from build123d import *

# Parameters (mm, degrees)
F0_R     = 8.5
F0_R_2   = 6.6901913145
F1_DEPTH = 25


# Not quite as in the source:
# - a feature names something its author has since deleted; it is built from what else it names


with BuildPart() as f1:
    # F0 (on Top) → F1 (new body)
    with BuildSketch(Plane.XY):
        with BuildLine():
            Line((147.8986507368, 41.0247598798), (-12.1013492632, 41.0247598798))
            ThreePointArc((-12.1013492632, 41.0247598798), (-33.5643369753, 37.6297800364), (-12.1013492632, 34.2348001929))
            Line((-12.1013492632, 34.2348001929), (-12.1013492632, 35.5247598798))
            Line((-12.1013492632, 35.5247598798), (147.8986507368, 35.5247598798))
            ThreePointArc((147.8986507368, 35.5247598798), (164.0425617184, 38.1300025139), (147.8986507368, 40.735245148))
            Line((147.8986507368, 40.735245148), (147.8986507368, 41.0247598798))
        make_face()
        with Locations((-22.5643369753, 37.6297800364)):
            Circle(F0_R, mode=Mode.SUBTRACT)
        with Locations((155.7603941795, 38.1300025139)):
            Circle(F0_R_2, mode=Mode.SUBTRACT)
    extrude(amount=F1_DEPTH)


solid = f1.part
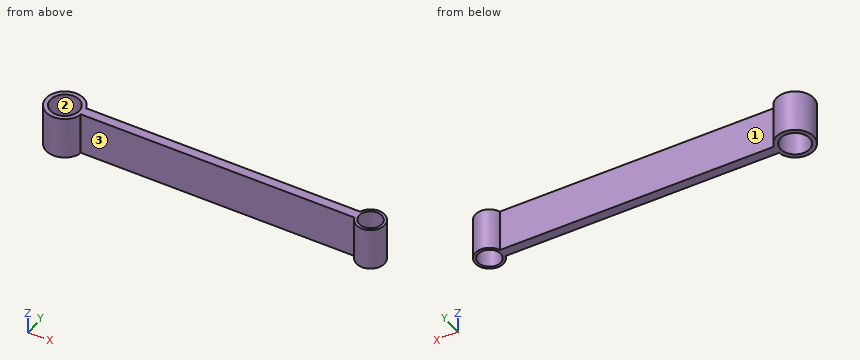
Build history of the part. All positions in model axes, mm. Face numbers are marked on the shaded views. A direction names the side the tool comes from. Coordinates: 2 decimals unless noted, no trailing zeros. Write each loop counter-clockwise with the first axis right and the second up, starting at its lowest first coordinate (ties: lowest second). Pieces come first, ordered by that corner, then holes.
(1) Pin check, flat tips, straight feed: pin 1 Ø7.5 at (x, z) = (63, 9) entering from +Y; pin 2 Ø4 at (x, z) = (-12, 3) entering from +Y; pin 3 Ø6 at (y, z) = (44, 11) entering from -X. Stop position of each tip, or through.
(2) Drill centre lines: line 1 (Y direction, x = 156, z = 17.75); line 2 (X direction, y = 36, z = 4.5); line 3 (X direction, y = 33.5, z = 4) (3 decimals). Where is each one in solid material? Low to high.
(3) 3-axis set-ups, long thin cutter, end or side, ignore diameter. For the marked faces 1, 2 and 3: which of +Z, -Z, +X, -X, +Y, -Y reach the whole face in a straight line?
(4) Cut at B-B on y = 42.75. List the corners of the cut face in (x, z), and give its area (3 significant figures).
(5) Cut at A-A on x = -20.5. List the corners of the cut face in (y, z).
(6) Cut at C-C on z = 4.5. List the corners of the cut face in (x, y), and give its area (3 significant figures).
(7) Cut at D-D on x = 26.5. List the corners of the cut face in (y, z).
Working result:
1. pin 1: stops at y = 41.02
1. pin 2: stops at y = 44.53
1. pin 3: stops at x = -33.04
2. line 1: y = 29.85 to 31.44, 44.82 to 46.41
2. line 2: x = -33.44 to -30.91, -14.22 to 149.42, 162.1 to 163.76
2. line 3: x = -32.76 to -29.994, -15.135 to -12.369, 148.893 to 150.931, 160.59 to 162.628
3. face 1: +Z, -Z, +Y
3. face 2: +Z, -Z
3. face 3: +Z, -Z, -Y
4. outline: (-32.3, 0) - (-29.35, 0) - (-29.35, 25) - (-32.3, 25) - close; (-15.78, 0) - (-12.83, 0) - (-12.83, 25) - (-15.78, 25) - close; (148.89, 0) - (150.92, 0) - (150.92, 25) - (148.89, 25) - close; (160.6, 0) - (162.63, 0) - (162.63, 25) - (160.6, 25) - close
4. area: 249 mm2
5. outline: (26.83, 0) - (29.38, 0) - (29.38, 25) - (26.83, 25) - close; (45.88, 0) - (48.43, 0) - (48.43, 25) - (45.88, 25) - close
6. outline: (-12.1, 34.23) - (-12.1, 35.52) - (147.9, 35.52) arc R8.28 ccw (long way) to (147.9, 40.74) - (147.9, 41.02) - (-12.1, 41.02) arc R11 ccw (long way) to start; hole circle Ø17 at (-22.56, 37.63); hole circle Ø13.38 at (155.76, 38.13)
6. area: 1,100 mm2
7. outline: (35.52, 0) - (41.02, 0) - (41.02, 25) - (35.52, 25) - close
